Could you check a few things on this model? Use its own coordinates, in mm. A direction names the side the tool comes from. Coordinates: 2 decimals unless noted, no trailing zeros. Order: outer loops, then holes, each group sorted by start corner. A loop starts at its lowest first (then second) coordinate and runs counter-clockwise, first axis right, second up. Notation, with made-up numbers: (28.25, 24) - (46.25, 24) arc R34 ccw to (46.25, 57) - close; hole circle Ø9 at (12, 1). An arc over 180 degrees is marked (long way). Answer as a JSON object with one key per item and string values. Group by question number.
(1) Please list where these lines run through material, in increasing order: probe 1 along Z at (x, y) = (2.5, 10); probe 2 along Y at (x, z) = (14, -19); probe 3 along Z at (x, y) = (15.25, 23).
(2) Imagine slicing it at B-B, the plane x = 12.75. Write out the boundary of the cut face in (y, z).
(3) Which directions (+Z, -Z, +X, -X, +Y, -Y) give clear straight access to the entire face, cutting with the end or side of a thin tool? Please do faces 1 (the flat face through (9, 79, 45)), 2 (the cylindrical face through (9.93, 46.31, 10.79)).
(4) We'd pull the mould along Y, two halves only. Please class faces 3 (the flat face through (9, 160, -1)), 4 (the cylindrical face through (9.93, 46.31, -12.71)), 5 (the flat face through (9, 79, -45)): pulls with the +Y half, pulls with the -Y half, needs draft (parallel to the pull), parting line crosses it, or undercut.
(5) Imagine slicing it at D-D, the plane y = 63.5. Write out the boundary of the cut face in (x, z).
(6) Will these pins go through, and if not, where does the flat tip stop? P1, Ø2.5, axis at y = 21, z = 12.5, coming from the +X side; P2, Ø3, axis at y = 55, z = 0, coming from the -X side; P3, Ø4, axis at y = 12.5, z = -29, coming from the +X side; P4, Ø7.5, axis at y = 58, z = 9.5, coming from the +X side.
(7) Imagine slicing it at A-A, the plane z = 0. Write out the boundary of the cut face in (x, y), and give its area (3 significant figures).
(8) Imagine slicing it at C-C, the plane y = 106.5. Write out the boundary of the cut face in (x, z).
from build123d import *

# Parameters (mm, degrees)
SKETCH_W        = 160
SKETCH_H        = 90
PAD_DEPTH       = 5
SKETCH001_R     = 7
PAD001_DEPTH    = 3
SKETCH002_R     = 2.5
PAD002_DEPTH    = 10
SKETCH003_R     = 0.8
PAD003_DEPTH    = 2.5
SKETCH004_R     = 1.4
POCKET_DEPTH    = 8
SKETCH005_W     = 25
SKETCH005_H     = 50
PAD004_DEPTH    = 2
SKETCH006_R     = 2.65
POCKET001_DEPTH = 7
CHAMFER_SIZE    = 1
CHAMFER001_SIZE = 1
SKETCH007_W     = 160
SKETCH007_H     = 90
SKETCH007_W_2   = 155
SKETCH007_H_2   = 85
PAD005_DEPTH    = 13
SKETCH008_W     = 12
SKETCH008_H     = 7
POCKET002_DEPTH = 5


with BuildPart() as part:
    # Sketch → Pad (new body)
    with BuildSketch(Plane.YZ):
        with Locations((80, 0)):
            Rectangle(SKETCH_W, SKETCH_H)
    extrude(amount=PAD_DEPTH)

    # Sketch001 (on Face6 of Pad) → Pad001 (join)
    with BuildSketch(Plane.YZ.offset(5)):
        with Locations((10, 31.75)):
            Circle(SKETCH001_R)
        with Locations((10, -31.75)):
            Circle(SKETCH001_R)
    extrude(amount=PAD001_DEPTH)

    # Sketch002 (on Face5 of Pad001) → Pad002 (join)
    with BuildSketch(Plane.YZ.offset(5)):
        with Locations((20, 11.75)):
            Circle(SKETCH002_R)
        with Locations((44, 11.75)):
            Circle(SKETCH002_R)
        with Locations((20, -11.75)):
            Circle(SKETCH002_R)
        with Locations((44, -11.75)):
            Circle(SKETCH002_R)
    extrude(amount=PAD002_DEPTH)

    # Sketch003 (on Face13 of Pad002) → Pad003 (join)
    with BuildSketch(Plane.YZ.offset(15)):
        with Locations((44, 11.75)):
            Circle(SKETCH003_R)
        with Locations((20, 11.75)):
            Circle(SKETCH003_R)
        with Locations((20, -11.75)):
            Circle(SKETCH003_R)
        with Locations((44, -11.75)):
            Circle(SKETCH003_R)
    extrude(amount=PAD003_DEPTH)

    # Sketch004 (on Face16 of Pad003) → Pocket (cut)
    with BuildSketch(Plane.YZ.offset(8)):
        with Locations((10, 31.75)):
            Circle(SKETCH004_R)
        with Locations((10, -31.75)):
            Circle(SKETCH004_R)
    extrude(amount=-POCKET_DEPTH, mode=Mode.SUBTRACT)

    # Sketch005 (on Face5 of Pocket) → Pad004 (join)
    with BuildSketch(Plane.YZ.offset(5)):
        with Locations((62.5, 0)):
            Rectangle(SKETCH005_W, SKETCH005_H)
    extrude(amount=PAD004_DEPTH)

    # Sketch006 (on Face21 of Pad004) → Pocket001 (cut)
    with BuildSketch(Plane.YZ.offset(7)):
        with Locations((55, 0)):
            Circle(SKETCH006_R)
        with Locations((70, 0)):
            Circle(SKETCH006_R)
    extrude(amount=-POCKET001_DEPTH, mode=Mode.SUBTRACT)

    # Chamfer
    chamfer_edges = [part.edges().sort_by_distance(p)[0] for p in [
        (0, 52.35, 0),
    ]]
    chamfer(chamfer_edges, length=CHAMFER_SIZE)

    # Chamfer001
    chamfer001_edges = [part.edges().sort_by_distance(p)[0] for p in [
        (0, 67.35, 0),
    ]]
    chamfer(chamfer001_edges, length=CHAMFER001_SIZE)

    # Sketch007 (on Face12 of Chamfer001) → Pad005 (join)
    with BuildSketch(Plane.YZ.offset(5)):
        with Locations((80, 0)):
            Rectangle(SKETCH007_W, SKETCH007_H)
        with Locations((80, 0)):
            Rectangle(SKETCH007_W_2, SKETCH007_H_2, mode=Mode.SUBTRACT)
    extrude(amount=PAD005_DEPTH)

    # Sketch008 (on Face42 of Pad005) → Pocket002 (cut)
    with BuildSketch(Plane.YX.offset(45)):
        with Locations((106, 12.5)):
            Rectangle(SKETCH008_W, SKETCH008_H)
    extrude(amount=-POCKET002_DEPTH, mode=Mode.SUBTRACT)


solid = part.part
Result set:
{
 "1": {"probe 1": "z = -45 to -33.15, -30.35 to 30.35, 33.15 to 45", "probe 2": "y = 0 to 2.5, 157.5 to 160", "probe 3": "z = -45 to -42.5, 42.5 to 45"},
 "2": {"outline": "(0, -45) - (100, -45) - (100, -42.5) - (2.5, -42.5) - (2.5, 42.5) - (157.5, 42.5) - (157.5, -42.5) - (112, -42.5) - (112, -45) - (160, -45) - (160, 45) - (0, 45) - close; circle Ø5 at (20, -11.75); circle Ø5 at (20, 11.75); circle Ø5 at (44, -11.75); circle Ø5 at (44, 11.75)"},
 "3": {"face 1": "+Z, +X, -X, +Y, -Y", "face 2": "+X"},
 "4": {"face 3": "pulls with the +Y half", "face 4": "undercut", "face 5": "needs draft"},
 "5": {"outline": "(0, -45) - (18, -45) - (18, -42.5) - (5, -42.5) - (5, -25) - (7, -25) - (7, 25) - (5, 25) - (5, 42.5) - (18, 42.5) - (18, 45) - (0, 45) - close"},
 "6": {"P1": "stops at x = 17.5", "P2": "passes through", "P3": "stops at x = 8", "P4": "stops at x = 7"},
 "7": {"outline": "(0, 0) - (18, 0) - (18, 2.5) - (5, 2.5) - (5, 50) - (7, 50) - (7, 52.35) - (1, 52.35) - (0, 51.35) - close; (0, 58.65) - (1, 57.65) - (7, 57.65) - (7, 67.35) - (1, 67.35) - (0, 66.35) - close; (0, 73.65) - (1, 72.65) - (7, 72.65) - (7, 75) - (5, 75) - (5, 157.5) - (18, 157.5) - (18, 160) - (0, 160) - close", "area": "839 mm^2"},
 "8": {"outline": "(0, -45) - (9, -45) - (9, -42.5) - (5, -42.5) - (5, 42.5) - (18, 42.5) - (18, 45) - (0, 45) - close; (16, -45) - (18, -45) - (18, -42.5) - (16, -42.5) - close"}
}
